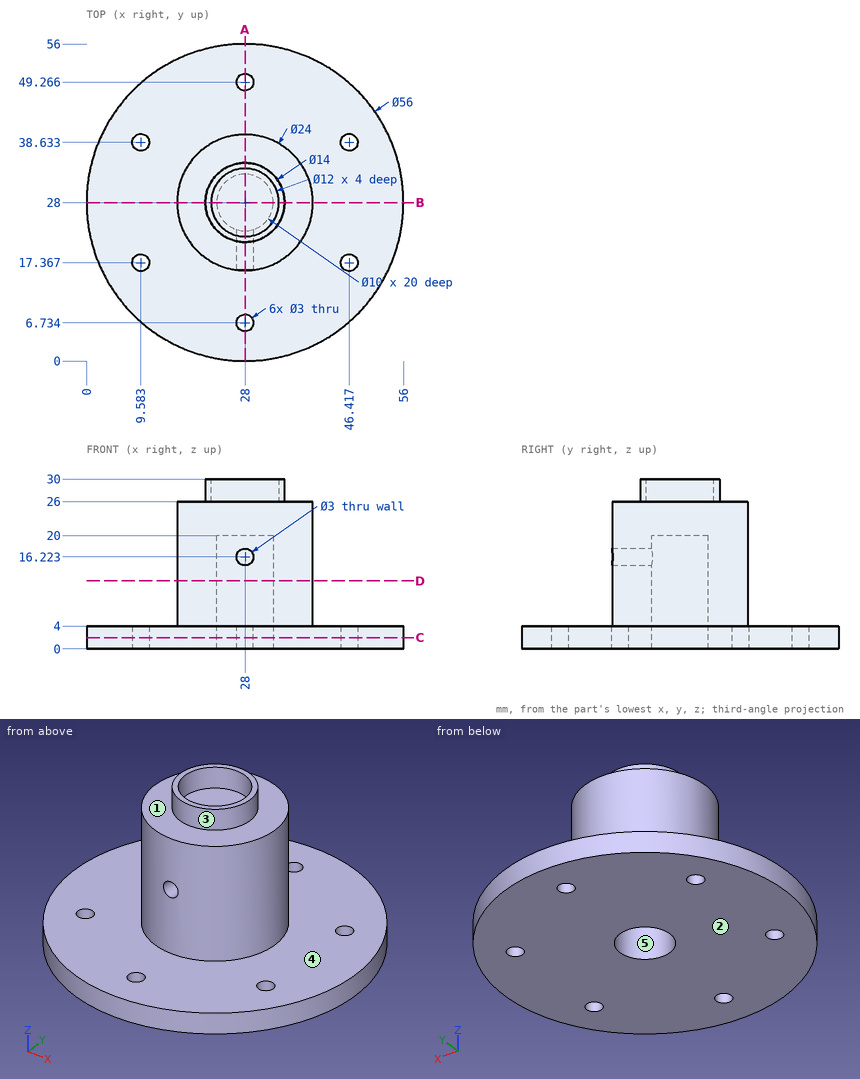
Check sheet for the drawn part. Datum: minimum x, y, z corner. Units: mm. A direction names the side the tool comes from. Round coordinates to 2 decimals unless told otherwise and drop trailing zeros. Order: outer loops, then holes, each group sorted by start corner. A loop starts at its lowest first (then second) coordinate and runs counter-clockwise, first axis right, second up.
1. Access from +Z, -Z, +X, -X, +Y, -Y to the whole of each face (thin tool, end or side, straight path). Record for the marked faces 1 and 2.
Final values:
face 1: +Z
face 2: -Z, +X, -X, +Y, -Y
2. Release check for a two-part mould opening along Y. For the marked faces 3, 4 and 5 record: +Y half, -Y half, draft (parallel to the pull), parting line (faces both ways), or undercut.
Final values:
face 3: parting line
face 4: draft
face 5: undercut
3. Section check A-A on x = 28. State how many separate pieces and enclosed holes the cut face has, then the cut area to 3 significant figures.
Final values:
separate pieces: 4
enclosed holes: 0
area: 515 mm2
4. Section check D-D on z = 12. Record the cut outline in (x, y).
Final values:
outline: circle Ø24 at (28, 28); hole circle Ø10 at (28, 28)
5. Go/stop test with flat-tipped pins: P1, Ø1.8, axis at x = 28, z = 16.22, coming from the +Y side; P2, Ø10, axis at x = 22.5, z = 3.5, coming from the -Y side; P3, Ø6, axis at x = 28, y = 28, coming from the +Z side. Record where each tip stops, or that it passes through.
Final values:
P1: stops at y = 40
P2: stops at y = 0
P3: stops at z = 26
6. Section check C-C on z = 2. Record the cut outline in (x, y) (1 decimal).
Final values:
outline: circle Ø56 at (28, 28); hole circle Ø3 at (9.6, 17.4); hole circle Ø3 at (9.6, 38.6); hole circle Ø10 at (28, 28); hole circle Ø3 at (28, 6.7); hole circle Ø3 at (28, 49.3); hole circle Ø3 at (46.4, 17.4); hole circle Ø3 at (46.4, 38.6)
7. Thickness scan on L1, parallel to Y at x = 28, z = 1.45 (1 decimal); L2, parallel to Z at x = 46, y = 43.5; L3, parallel to Z at x = 25.5, y = 28. Record the ranges inside material, lowest first.
Final values:
L1: y = 0 to 5.2, 8.2 to 23, 33 to 47.8, 50.8 to 56
L2: z = 0 to 4
L3: z = 20 to 26
8. Section check B-B on y = 28. Record the cut outline in (x, z), then the cut area to 3 significant figures.
Final values:
outline: (0, 0) - (23, 0) - (23, 20) - (33, 20) - (33, 0) - (56, 0) - (56, 4) - (40, 4) - (40, 26) - (35, 26) - (35, 30) - (34, 30) - (34, 26) - (22, 26) - (22, 30) - (21, 30) - (21, 26) - (16, 26) - (16, 4) - (0, 4) - close
area: 560 mm2
